from build123d import *

# Parameters (mm, degrees)
EXTRUDE_1_DEPTH     = 5
SKETCH_4_R          = 3.35
CUT_EXTRUDE_1_DEPTH = 5


with BuildPart() as part:
    # 草图1 → 凸台-拉伸1 (new body)
    with BuildSketch(Plane.XY):
        with BuildLine():
            Line((33.882068439, 36.885004962), (7.846534534, 10.849471056))
            Line((7.846534534, 10.849471056), (-8.011329843, 10.849471056))
            Line((-8.011329843, 10.849471056), (-34.046863749, 36.885004962))
            ThreePointArc((-34.046863749, 36.885004962), (-41.117931561, 36.885004962), (-41.117931561, 29.81393715))
            Line((-41.117931561, 29.81393715), (-17.582397655, 6.278403244))
            Line((-17.582397655, 6.278403244), (-17.582397655, -14.579461132))
            Line((-17.582397655, -14.579461132), (-41.117931561, -38.114995038))
            ThreePointArc((-41.117931561, -38.114995038), (-41.117931561, -45.18606285), (-34.046863749, -45.18606285))
            Line((-34.046863749, -45.18606285), (-8.011329843, -19.150528944))
            Line((-8.011329843, -19.150528944), (7.846534534, -19.150528944))
            Line((7.846534534, -19.150528944), (33.882068439, -45.18606285))
            ThreePointArc((33.882068439, -45.18606285), (40.953136251, -45.18606285), (40.953136251, -38.114995038))
            Line((40.953136251, -38.114995038), (17.417602345, -14.579461132))
            Line((17.417602345, -14.579461132), (17.417602345, 6.278403244))
            Line((17.417602345, 6.278403244), (40.953136251, 29.81393715))
            ThreePointArc((40.953136251, 29.81393715), (40.953136251, 36.885004962), (33.882068439, 36.885004962))
        make_face()
    extrude(amount=EXTRUDE_1_DEPTH)

    # 草图4 → 切除-拉伸1 (cut)
    with BuildSketch(Plane.XY.offset(5)):
        with Locations((-37.582397655, 33.349471056)):
            Circle(SKETCH_4_R)
        with Locations((37.417602345, 33.349471056)):
            Circle(SKETCH_4_R)
        with Locations((37.417602345, -41.650528944)):
            Circle(SKETCH_4_R)
        with Locations((-37.582397655, -41.650528944)):
            Circle(SKETCH_4_R)
    extrude(amount=-CUT_EXTRUDE_1_DEPTH, mode=Mode.SUBTRACT)


solid = part.part
Build history of the part. All positions in model axes, mm. A direction names the side the tool comes from. Coordinates: 2 decimals unless noted, no trailing zeros. Write each loop counter-clockwise with the first axis right and the second up, starting at its lowest first coordinate (ties: lowest second). Pieces come first, ordered by that corner, then holes.
(1) 3-axis set-ups, long thin cutter, end or side, ignore diameter. For faces 1 (the flat face through (29.35, -26.51, 2.46)), 2 (the flat face through (-17.582, -4, 2)), 3 (the flat face through (-20.847, 23.685, 2.465)), 4 (the flat face through (0, -19.151, 2)): which of +Z, -Z, +X, -X, +Y, -Y reach the whole face in a straight line?
(2) Mould opens along X. For faces 5 (the flat face through (-29.185, -26.182, 2.465)), 6 (the flat face through (0, -4, 0)), 7 (the cylindrical face through (39.219, 36.174, 2.535)) say: pulls with the +X half, pulls with the -X half, needs draft (parallel to the pull), parting line crosses it, or undercut.
(3) Cut at D-D on x = 29. List the corners of the cut face in (y, z).
(4) Pin check, flat tips, straight feed: pin 1 Ø6 at (x, y) = (-10.5, -21) entering from -Z; pin 2 Ø1.5 at (y, z) = (-2, 2.5) entering from +X; pin 3 Ø2 at (x, z) = (27.5, 2) entering from +Y; pin 4 Ø1 at (x, z) = (7.5, 1.5) entering from +Y. Stop position of each tip, or through.
(5) Cut at A-A on y = -40. List the corners of the cut face in (x, z).
(6) Cut at B-B on z = 2.6. List the corners of the cut face in (x, y) (3 decimals).
(7) Cut at C-C on x = -37. List the corners of the cut face in (y, z), and give its area (3 significant figures).
(8) Drill centre lines: line 1 (X direction, y = -40, z = 1.2); line 2 (Y direction, x = -37, z = 2.65); line 3 (X direction, y = -10.5, z = 3.25). Where is each one in solid material? Low to high.
Working result:
1. face 1: +Z, -Z, +X
1. face 2: +Z, -Z, -X
1. face 3: +Z, -Z, +Y
1. face 4: +Z, -Z, -Y
2. face 5: pulls with the -X half
2. face 6: needs draft
2. face 7: undercut
3. outline: (-40.3, 0) - (-26.16, 0) - (-26.16, 5) - (-40.3, 5) - close; (17.86, 0) - (32, 0) - (32, 5) - (17.86, 5) - close
4. pin 1: stops at z = 0
4. pin 2: stops at x = 17.42
4. pin 3: stops at y = 31.5
4. pin 4: stops at y = 11
5. outline: (-42.3, 0) - (-40.5, 0) - (-40.5, 5) - (-42.3, 5) - close; (-34.67, 0) - (-28.86, 0) - (-28.86, 5) - (-34.67, 5) - close; (28.7, 0) - (34.5, 0) - (34.5, 5) - (28.7, 5) - close; (40.33, 0) - (42.14, 0) - (42.14, 5) - (40.33, 5) - close
6. outline: (-41.118, -38.115) arc R5 ccw to (-34.047, -45.186) - (-8.011, -19.151) - (7.847, -19.151) - (33.882, -45.186) arc R5 ccw to (40.953, -38.115) - (17.418, -14.579) - (17.418, 6.278) - (40.953, 29.814) arc R5 ccw to (33.882, 36.885) - (7.847, 10.849) - (-8.011, 10.849) - (-34.047, 36.885) arc R5 ccw to (-41.118, 29.814) - (-17.582, 6.278) - (-17.582, -14.579) - close; hole circle Ø6.7 at (-37.582, -41.651); hole circle Ø6.7 at (-37.582, 33.349); hole circle Ø6.7 at (37.418, -41.651); hole circle Ø6.7 at (37.418, 33.349)
7. outline: (-46.62, 0) - (-44.95, 0) - (-44.95, 5) - (-46.62, 5) - close; (-38.35, 0) - (-34, 0) - (-34, 5) - (-38.35, 5) - close; (25.7, 0) - (30.05, 0) - (30.05, 5) - (25.7, 5) - close; (36.65, 0) - (38.32, 0) - (38.32, 5) - (36.65, 5) - close
7. area: 60.2 mm2
8. line 1: x = -42.3 to -40.5, -34.67 to -28.86, 28.7 to 34.5, 40.33 to 42.14
8. line 2: y = -46.62 to -44.95, -38.35 to -34, 25.7 to 30.05, 36.65 to 38.32
8. line 3: x = -17.58 to 17.42
